Autodesk Inventor part; units mm, degrees
ref_plane "YZ Plane" through (0, 0, 0) normal (1, 0, 0) x (0, 1, 0)
ref_plane "XZ Plane" through (0, 0, 0) normal (0, 1, 0) x (-1, 0, 0)
ref_plane "XY Plane" through (0, 0, 0) normal (0, 0, 1) x (1, 0, 0)
sketch "Sketch1" plane through (0, 0, 0) normal (0, 0, 1) x (1, 0, 0)
  line L0 (0, 0) -> (72.136, 0)
  line L1 (72.136, 0) -> (72.136, 59.69)
  line L2 (72.136, 59.69) -> (0, 59.69)
  line L3 (0, 59.69) -> (0, 0)
  dimension "d0" = 59.69
  dimension "d1" = 72.136
extrude "Extrusion1" add sketch "Sketch1" along normal blind 21.844
sketch "Sketch2" plane through (0, 0, 21.844) normal (0, 0, 1) x (1, 0, 0)
  line L0 (3.048, 56.642) -> (69.088, 56.642)
  line L1 (69.088, 56.642) -> (69.088, 3.048)
  line L2 (69.088, 3.048) -> (3.048, 3.048)
  line L3 (3.048, 3.048) -> (3.048, 56.642)
  line L4 (72.136, 59.69) -> (0, 59.69)
  line L5 (72.136, 0) -> (72.136, 59.69)
  line L6 (0, 0) -> (72.136, 0)
  line L7 (0, 59.69) -> (0, 0)
  dimension "d4" = 3.048
  dimension "d5" = 3.048
  dimension "d6" = 3.048
  dimension "d7" = 3.048
extrude "Extrusion2" cut sketch "Sketch2" against normal blind 15.24 contours L0 L1 L2 L3
sketch "Sketch3" plane through (0, 0, 6.604) normal (0, 0, 1) x (1, 0, 0)
  line L0 (15.113, 45.72) -> (30.607, 45.72)
  line L1 (30.607, 45.72) -> (30.607, 51.689)
  line L2 (30.607, 51.689) -> (15.113, 51.689)
  line L3 (15.113, 51.689) -> (15.113, 45.72)
  line L4 (3.048, 56.642) -> (69.088, 56.642)
  line L5 (3.048, 3.048) -> (3.048, 56.642)
  circle A0 centre (23.622, 33.274) radius 2.794
  circle A1 centre (27.178, 11.5062) radius 2.794
  point P0 (0, 0)
  dimension "d10" = 5.969
  dimension "d11" = 15.494
  dimension "d12" = 4.953
  dimension "d13" = 12.065
  dimension "d14" = 5.588
  dimension "d15" = 5.588
  dimension "d17" = 24.13
  dimension "d18" = 20.574
  dimension "d21" = 23.368
  dimension "d22" = 45.1358
extrude "Extrusion3" cut sketch "Sketch3" against normal blind 1.778
sketch "Sketch4" plane through (0, 0, 21.844) normal (0, 0, 1) x (1, 0, 0)
  point P0 (0, 0)
sketch "Sketch5" plane through (0, 0, 21.844) normal (0, 0, 1) x (1, 0, 0)
  line L0 (-2.54, -2.54) -> (74.676, -2.54)
  line L1 (74.676, -2.54) -> (74.676, 62.23)
  line L2 (74.676, 62.23) -> (-2.54, 62.23)
  line L3 (-2.54, 62.23) -> (-2.54, -2.54)
  line L4 (72.136, 0) -> (72.136, 59.69)
  line L5 (72.136, 59.69) -> (0, 59.69)
  line L6 (0, 59.69) -> (0, 0)
  line L7 (0, 0) -> (72.136, 0)
  line L8 (0, 0) -> (72.136, 0)
  line L9 (72.136, 0) -> (72.136, 59.69)
  line L10 (72.136, 59.69) -> (0, 59.69)
  line L11 (0, 59.69) -> (0, 0)
  dimension "d23" = 2.54
  dimension "d24" = 2.54
  dimension "d25" = 2.54
  dimension "d26" = 2.54
extrude "Extrusion4" add sketch "Sketch5" against normal blind 21.844
sketch "Sketch6" plane through (0, 0, 21.844) normal (0, 0, 1) x (1, 0, 0)
  line L0 (-0.762, -0.762) -> (72.898, -0.762)
  line L1 (72.898, -0.762) -> (72.898, 60.452)
  line L2 (72.898, 60.452) -> (-0.762, 60.452)
  line L3 (-0.762, 60.452) -> (-0.762, -0.762)
  line L4 (3.048, 3.048) -> (3.048, 56.642)
  line L5 (3.048, 56.642) -> (69.088, 56.642)
  line L6 (69.088, 56.642) -> (69.088, 3.048)
  line L7 (69.088, 3.048) -> (3.048, 3.048)
  point P0 (0, 0)
  dimension "d29" = 3.81
  dimension "d30" = 3.81
  dimension "d31" = 3.81
  dimension "d32" = 3.81
extrude "Extrusion5" cut sketch "Sketch6" against normal blind 15.24
sketch "Sketch7" plane through (0, 0, 21.844) normal (0, 0, 1) x (1, 0, 0)
  point P0 (0, 0)
sketch "Sketch8" plane through (0, 0, 21.844) normal (0, 0, 1) x (1, 0, 0)
  line L0 (74.676, -2.54) -> (-2.54, -2.54)
  line L1 (-2.54, -2.54) -> (74.676, -2.54)
  line L2 (74.676, -2.54) -> (74.676, 62.23)
  line L3 (74.676, 62.23) -> (-2.54, 62.23)
  line L4 (-2.54, 62.23) -> (-2.54, -2.54)
  line L5 (-7.62, -7.62) -> (79.756, -7.62)
  line L6 (79.756, -7.62) -> (79.756, 67.31)
  line L7 (79.756, 67.31) -> (-7.62, 67.31)
  line L8 (-7.62, 67.31) -> (-7.62, -7.62)
  point P0 (0, 0)
  dimension "d35" = 5.08
  dimension "d36" = 5.08
  dimension "d37" = 5.08
  dimension "d38" = 5.08
extrude "Extrusion6" add sketch "Sketch8" against normal blind 21.844
sketch "Sketch10" plane through (0, 0, 21.844) normal (0, 0, 1) x (1, 0, 0)
  point P0 (0, 0)
sketch "Sketch15" plane through (0, 0, 21.844) normal (0, 0, 1) x (1, 0, 0)
  line L0 (72.898, -0.762) -> (-0.762, -0.762)
  line L1 (-0.762, 60.452) -> (72.898, 60.452)
  line L2 (-0.762, -0.762) -> (72.898, -0.762)
  line L3 (72.898, -0.762) -> (72.898, 60.452)
  line L4 (72.898, 60.452) -> (-0.762, 60.452)
  line L5 (-0.762, 60.452) -> (-0.762, -0.762)
  line L6 (70.358, 57.912) -> (1.778, 57.912)
  line L7 (1.778, 57.912) -> (1.778, 1.778)
  line L8 (1.778, 1.778) -> (70.358, 1.778)
  line L9 (70.358, 1.778) -> (70.358, 57.912)
  point P0 (0, 0)
  dimension "d63" = 2.54
  dimension "d64" = 2.54
  dimension "d65" = 2.54
  dimension "d66" = 2.54
extrude "Extrusion8" add sketch "Sketch15" against normal blind 15.24
sketch "Sketch16" plane through (0, 0, 21.844) normal (0, 0, 1) x (1, 0, 0)
  line L0 (10.922, -4.572) -> (61.214, -4.572)
  line L1 (76.2, 10.414) -> (76.2, 49.276)
  line L2 (61.214, 64.262) -> (10.922, 64.262)
  line L3 (-4.064, 49.276) -> (-4.064, 10.414)
  line L4 (1.778, 57.912) -> (70.358, 57.912)
  line L5 (70.358, 1.778) -> (1.778, 1.778)
  line L6 (1.778, 1.778) -> (1.778, 57.912)
  line L7 (70.358, 57.912) -> (70.358, 1.778)
  line L8 (1.778, 57.912) -> (1.778, 1.778)
  line L9 (70.358, 1.778) -> (70.358, 57.912)
  line L10 (1.778, 1.778) -> (70.358, 1.778)
  line L11 (70.358, 1.778) -> (70.358, 57.912)
  line L12 (70.358, 57.912) -> (1.778, 57.912)
  line L13 (1.778, 57.912) -> (1.778, 1.778)
  arc A0 (-4.064, 10.414) -> (10.922, -4.572) centre (10.922, 10.414) ccw
  arc A1 (10.922, 64.262) -> (-4.064, 49.276) centre (10.922, 49.276) ccw
  arc A2 (76.2, 49.276) -> (61.214, 64.262) centre (61.214, 49.276) ccw
  arc A3 (61.214, -4.572) -> (76.2, 10.414) centre (61.214, 10.414) ccw
  point P0 (0, 0)
  dimension "d69" = 6.35
  dimension "d70" = 6.35
  dimension "d71" = 5.842
  dimension "d72" = 5.842
  dimension "d73" = 14.986
extrude "Extrusion9" cut sketch "Sketch16" against normal blind 15.24
fillet "Fillet2" radius 14.732 4 edges at (79.756, 67.31, 10.922) (79.756, -7.62, 10.922) (-7.62, 67.31, 10.922) (-7.62, -7.62, 10.922)
sketch "Sketch17" plane through (0, 0, 0) normal (0, 0, -1) x (-1, 0, 0)
  line L0 (-94.7004, 78.8948) -> (24.3491, 78.8948)
  line L1 (24.3491, 78.8948) -> (24.3491, -15.2836)
  line L2 (24.3491, -15.2836) -> (-94.7004, -15.2836)
  line L3 (-94.7004, -15.2836) -> (-94.7004, 78.8948)
  point P0 (0, 0)
extrude "Extrusion10" cut sketch "Sketch17" against normal blind 2.5
properties part number "Bottom_Housing_K30"
Read the model definition and answer for the solid it produces. Units are mm, in the model's axes. A direction names the side the tool comes from. Give positions to 0.01 mm unless a question says otherwise; leave off trailing zeros. Write each loop counter-clockwise with the first axis right and the second up, starting at its lowest first coordinate (ties: lowest second). Pieces come first, ordered by that corner, then holes. Notation, with made-up numbers: (-21.5, 13) - (22.5, 13) arc R16 ccw to (22.5, 39) - close; hole circle Ø10 at (30, 87.25). An arc over 180 degrees is marked (long way). Return JSON: item names as keys, results as strings.
Q1. For faces 1 (the face through (75.555, -3.19, 12.037)), 2 (the face through (30.607, 49, 6)), determine the directions among +Z, -Z, +X, -X, +Y, -Y from which every point of the face is accessible in a straight line to the end or side of a thin tool.
Reply:
{"face 1": "+Z, -Z, +X, -Y", "face 2": "+Z"}
Q2. For a pull along X with two mould halves and no side action, classify faces 3 (the face through (-3.4, 62.9, 12)), 4 (the face through (36, 67.31, 12)), 5 (the face through (23, 51.689, 6)), 6 (the face through (75.326, 63.109, 12.037)) as released by +X, released by -X, zero draft, split by the parting line, or undercut.
Reply:
{"face 3": "released by -X", "face 4": "zero draft", "face 5": "undercut", "face 6": "released by +X"}
Q3. A cutting plane is placed at D-D, the plane y = 35. Determine the outline of the cut face in (x, z).
Reply:
{"outline": "(-7.62, 2.5) - (79.76, 2.5) - (79.76, 21.84) - (76.2, 21.84) - (76.2, 6.6) - (25.82, 6.6) - (25.82, 4.83) - (21.42, 4.83) - (21.42, 6.6) - (-4.06, 6.6) - (-4.06, 21.84) - (-7.62, 21.84) - close"}
Q4. Given P1, Ø3, axis at x = 24, y = 32, coming from the +Z side; P2, Ø3, axis at x = 23.5, y = 50, coming from the +Z side, each flat-ended and moving along its own axis, determine where each tip first touches the part or whether it passes through.
Reply:
{"P1": "z = 6.6", "P2": "z = 4.83"}
Q5. A cutting plane is placed at B-B, the plane y = 20. Determine the outline of the cut face in (x, z).
Reply:
{"outline": "(-7.62, 2.5) - (79.76, 2.5) - (79.76, 21.84) - (76.2, 21.84) - (76.2, 6.6) - (-4.06, 6.6) - (-4.06, 21.84) - (-7.62, 21.84) - close"}
Q6. A cutting plane is placed at A-A, the plane z = 15. Determine the outline of the cut face in (x, y), and give its area (3 significant figures).
Reply:
{"outline": "(-7.62, 7.11) arc R14.73 ccw to (7.11, -7.62) - (65.02, -7.62) arc R14.73 ccw to (79.76, 7.11) - (79.76, 52.58) arc R14.73 ccw to (65.02, 67.31) - (7.11, 67.31) arc R14.73 ccw to (-7.62, 52.58) - close; hole (-4.06, 10.41) arc R14.99 ccw to (10.92, -4.57) - (61.21, -4.57) arc R14.99 ccw to (76.2, 10.41) - (76.2, 49.28) arc R14.99 ccw to (61.21, 64.26) - (10.92, 64.26) arc R14.99 ccw to (-4.06, 49.28) - close", "area": "1,030 mm²"}
Q7. A cutting plane is placed at C-C, the plane x = 39.5. Determine the outline of the cut face in (y, z).
Reply:
{"outline": "(-7.62, 2.5) - (67.31, 2.5) - (67.31, 21.84) - (64.26, 21.84) - (64.26, 6.6) - (-4.57, 6.6) - (-4.57, 21.84) - (-7.62, 21.84) - close"}
Q8. Consider line 1 along Y through (x, z) = (17.5, 20.5); line 2 along X through (y, z) = (36, 9.5); line 3 along Z through (x, y) = (28, 61.5). Determine where each line is inside the solid, lowest interval first. Write a range as [from, to].
Reply:
{"line 1": "[-7.62, -4.57], [64.26, 67.31]", "line 2": "[-7.62, -4.06], [76.2, 79.76]", "line 3": "[2.5, 6.6]"}
